Can you work these out from the drawing? Everything is in mm from the part's minimum corner. Coordinates: 2 decimals unless noted, no trailing zeros. Loops run counter-clockwise (first coordinate to the right, second up) from the corner with the lowest first, then second, coordinate; pieces in that order, holes last. Notation, with made-up numbers: (53, -40) -> (74, -40) arc R18 ccw to (74, -32) -> close; hole circle Ø8 at (-4, 77.5). An arc over 180 degrees is marked (long way). One line per question, with ' | ' between items.
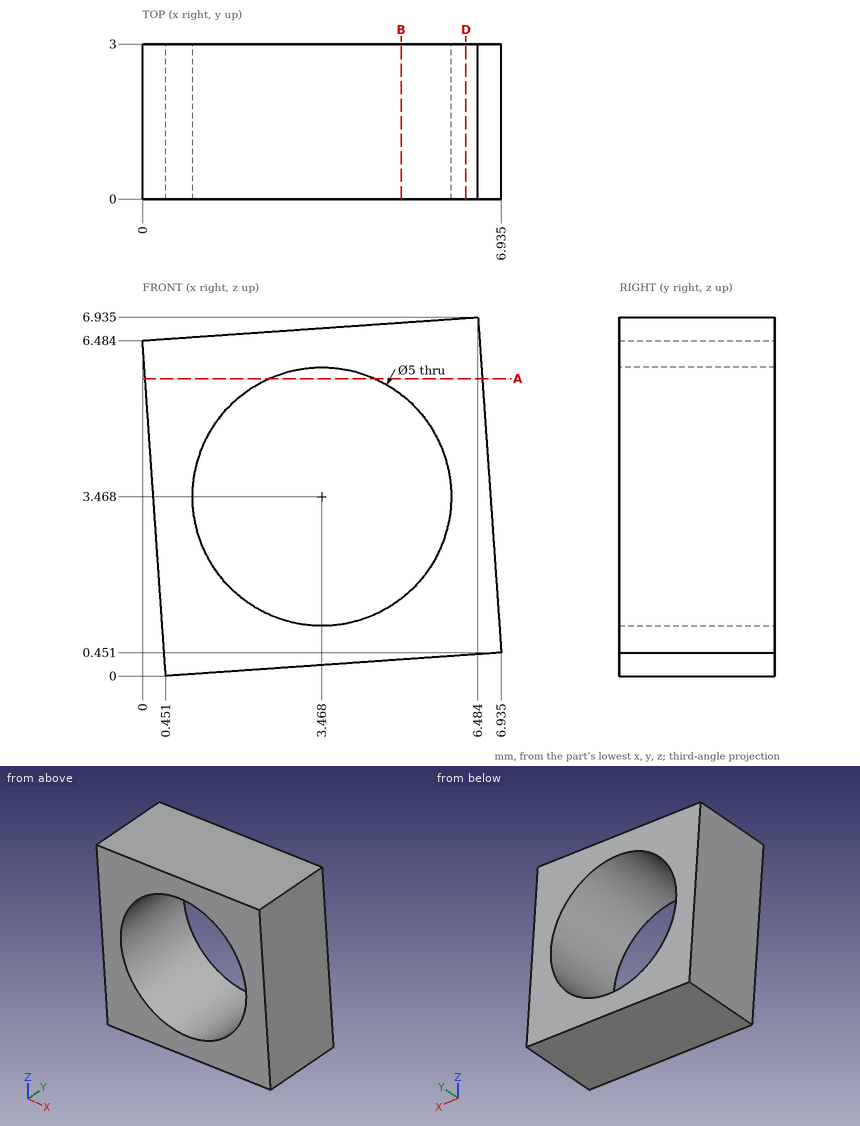
Q1. Imagine slicing it at B-B on x = 5. Write out the boundary of the cut face in (y, z).
Values follow:
outline: (0, 0.32) -> (3, 0.32) -> (3, 1.49) -> (0, 1.49) -> close; (0, 5.44) -> (3, 5.44) -> (3, 6.83) -> (0, 6.83) -> close
Q2. Imagine slicing it at A-A on z = 5.75. Write out the boundary of the cut face in (x, y), plus the area to 3 significant figures.
Values follow:
outline: (0.05, 0) -> (2.45, 0) -> (2.45, 3) -> (0.05, 3) -> close; (4.49, 0) -> (6.57, 0) -> (6.57, 3) -> (4.49, 3) -> close | area: 13.4 mm2
Q3. For pin 1 (1 mm diameter, centred on x = 3.5, z = 5, fed in from +Y); pin 2 (1 mm diameter, centred on y = 0.5, z = 5, fed in from -X); pin 3 (1 mm diameter, centred on x = 4, y = 2, fed in from -Z), each with a flat end and sliding along its axis, tell me the tip position at first contact or that it passes through.
Values follow:
pin 1: passes through | pin 2: stops at x = 0.07 | pin 3: stops at z = 0.21
Q4. Please list where these lines run through material, in increasing order: L1, parallel to Z at x = 3, y = 2; L2, parallel to X at y = 1, z = 5.25 (1 decimal); L3, parallel to X at y = 1.35, z = 1.5 (1 decimal). Write a range as [from, to].
Values follow:
L1: z = [0.18, 1.01], [5.92, 6.69] | L2: x = [0.1, 1.7], [5.2, 6.6] | L3: x = [0.3, 1.9], [5, 6.9]
Q5. Imagine slicing it at D-D on x = 6.25. Write out the boundary of the cut face in (y, z).
Values follow:
outline: (0, 0.4) -> (3, 0.4) -> (3, 6.92) -> (0, 6.92) -> close
